Could you check a few things on this model? Use its own coordinates, in mm. A direction names the side the tool comes from. Give positions to 0.01 mm unless a question says otherwise; leave off trailing zeros. Order: outer loops, then holes, each group sorted by start corner. A loop starts at its lowest first (then second) coordinate and runs counter-clockwise, first axis right, second up. Notation, with made-up numbers: M 22,-39 L 67,-39 A23 ccw 67,-27 Z; hole C 89.5,27 d2. An arc over 180 degrees is marked long. Use a Markdown table: item, result. Add a question column.
Item 1: If I drill on L1, parallel to X at y = 0, z = 47.5; L2, parallel to Y at x = 0, z = 71; L3, parallel to X at y = -1.25, z = 56.5, over which ranges is the centre line in solid material (lowest first)? Write a range as from..to.
Item 2: If we mould it in two halves opening along Y, with no side actions, what happens to faces 4 (the face through (6.269, 4.807, 88.79)), 5 (the face through (348.76, -9.42, 83.81))? For each: released by +Y, released by -Y, zero draft, split by the parting line, or undercut.
Item 3: Suppose I cut it at A-A on y = 0. Write out the boundary of the cut face in (x, z), plus the area to 3 significant figures.
Item 4: Suppose I cut it at B-B on z = 113.5. Write out the boundary of the cut face in (x, y), plus the area to 3 significant figures.
Item 5: For faces 1 (the face through (176.33, 3.639, 258.776)), 2 (the face through (357.535, -2.373, 86.484)), 3 (the face through (342.4, 2.8, 5.7)), which set-ups out of +Z, -Z, +X, -X, +Y, -Y let a thin tool reach every point of the face, with its end or its side?
Item 6: Suppose I cut it at C-C on x = 130.5. Write out the boundary of the cut face in (y, z).
Item 7: I'm going to push flat-ended pins straight in: pin 1 Ø6 at (x, y) = (182.5, -6) entering from +Z; pin 2 Ø4 at (y, z) = (7, 214.5) entering from -X; pin 3 Ø1.5 at (x, y) = (313, 6.5) entering from +Z. Where does each tip first touch, or does it pass through?
Solid Edge part; units mm, degrees
sketch "Sketch1" plane through (0, 0, 0) normal (0, -1, 0) x (1, 0, 0)
  line L0 (0, 0) -> (0, 170)
  arc A0 (0, 170) -> (80, 250) centre (80, 170) cw
  line L1 (80, 250) -> (270, 250)
  arc A1 (270, 250) -> (350, 170) centre (270, 170) cw
  line L2 (350, 170) -> (350, 0)
sketch "Sketch2" plane through (0, 0, 0) normal (0, 0, -1) x (-1, 0, 0)
  circle A0 centre (0, 0) radius 9.5
sweep "SweptProtrusion_1" add profiles "Sketch2" path "Sketch1"
shell "Thinwall_1" thickness 1.6 removed faces 4 at (6.5233, -6.1433, 0) at (343.4767, -6.1433, 0) at (6.5233, -6.1433, 0) at (343.4767, -6.1433, 0)
hole "Hole_1" at (0, 0, 0) direction (0, -1, 0) diameter 19 end through all both ways yes
hole "Hole1" at (350, 0, 0) direction (0, -1, 0) diameter 19 end through all both ways yes
properties material "Aluminum, 1060"
Findings below:
| question | item | result |
|---|---|---|
| 1 | L1 | x = -9.5..-7.9, 7.9..9.5, 340.5..342.1, 357.9..359.5 |
| 1 | L2 | y = -9.5..-7.9, 7.9..9.5 |
| 1 | L3 | x = -9.42..-7.8, 7.8..9.42, 340.58..342.2, 357.8..359.42 |
| 2 | face 4 | undercut |
| 2 | face 5 | split by the parting line |
| 3 | outline | M -9.5,0 A9.5 cw -7.9,5.28 L -7.9,170 A87.9 cw 80,257.9 L 270,257.9 A87.9 cw 357.9,170 L 357.9,5.28 A9.5 cw 359.5,0 L 359.5,170 A89.5 ccw 270,259.5 L 80,259.5 A89.5 ccw -9.5,170 Z; M 7.9,5.28 A9.5 cw 9.5,0 L 9.5,170 A70.5 cw 80,240.5 L 270,240.5 A70.5 cw 340.5,170 L 340.5,0 A9.5 cw 342.1,5.28 L 342.1,170 A72.1 ccw 270,242.1 L 80,242.1 A72.1 ccw 7.9,170 Z |
| 3 | area | 2,480 mm^2 |
| 4 | outline | C 0,0 d19; C 350,0 d19; hole C 0,0 d15.8; hole C 350,0 d15.8 |
| 4 | area | 175 mm^2 |
| 5 | face 1 | none |
| 5 | face 2 | -Z |
| 5 | face 3 | -Z, +Y, -Y |
| 6 | outline | C 0,250 d19; hole C 0,250 d15.8 |
| 7 | pin 1 | stops at z = 259.01 |
| 7 | pin 2 | stops at x = 3.6 |
| 7 | pin 3 | stops at z = 246.4 |
